Read the model definition and answer for the solid it produces. Units are mm, in the model's axes. Coordinates: 2 decimals unless noted, no trailing zeros. Order: outer loops, then holes, each group sorted by start corner. A loop starts at its lowest first (then second) coordinate and runs counter-clockwise, first axis right, second up. Notation, with made-up numbers: (-8, -12) -> (20, -12) arc R22 ccw to (20, 11) -> close; hole circle Ø2 at (83, 38). An arc over 180 degrees is marked (long way). Answer as a JSON object with one key per item and string values. Group by question number.
1) Given pin 1 (5.5 mm diameter, centred on y = 0, z = -48, fed in from +X); pin 2 (2 mm diameter, centred on x = 6.5, z = 40.5, fed in from -Y), each flat-ended and moving along its own axis, determine where each tip first touches the part or whether it passes through.
2) Consider L1, parallel to Z at x = 2.9, y = 0; L2, parallel to Z at x = 5.5, y = 0; L3, parallel to Y at x = 3.85, z = 0. Determine where each line is inside the solid, lowest interval first.
3) Section D-D on x = 8 is taken. Determine the outline of the cut face in (y, z).
4) Section C-C on y = 15 is taken. Determine the outline of the cut face in (x, z).
5) Section B-B on z = -24 is taken. Determine the outline of the cut face in (x, y), and give its area (3 significant figures).
6) Section A-A on y = 0 is taken. Determine the outline of the cut face in (x, z).
from build123d import *

# Parameters (mm, degrees)
F0_W            = 10
F0_H            = 17
F2_R            = 3.5
F3_DEPTH        = 10.001
F3_COPIES_COUNT = 6
F5_DEPTH        = 10.001
F6_R            = 39.5
F6_R_2          = 37
F7_DEPTH        = 5


# Not quite as in the source:
# - a pattern or mirror of a feature is missing from the dataset's text; its kind, count and spacing are read off the source's solid


with BuildPart() as f1:
    # F0 (on Front) → F1 (revolve)
    with BuildSketch(Plane.XZ):
        with Locations((5, 45.5)):
            Rectangle(F0_W, F0_H)
    revolve(axis=Axis((-28.7704151153, 0, 0), (-1, 0, 0)))

    # F2 (on face) → F3 (cut, through all)
    with BuildSketch(Plane(origin=(0, 0, 0), x_dir=(0, -1, 0), z_dir=(-1, 0, 0))):
        with Locations((41.5692193817, 24)):
            Circle(F2_R)
    f3 = extrude(amount=-F3_DEPTH, mode=Mode.SUBTRACT)

    # F3_copies: F3 ×6 about axis
    f3_copies_axis = Axis((0, 0, 0), (1, 0, 0))
    for i in range(1, F3_COPIES_COUNT):
        add(f3.rotate(f3_copies_axis, i * 360 / F3_COPIES_COUNT), mode=Mode.SUBTRACT)

    # F4 (on face) → F5 (cut, through all)
    with BuildSketch(Plane(origin=(0, 0, 0), x_dir=(0, -1, 0), z_dir=(-1, 0, 0))):
        with BuildLine():
            Line((-50, -20.3960780544), (-50, 20.3960780544))
            ThreePointArc((-50, 20.3960780544), (-54, 0), (-50, -20.3960780544))
        make_face()
        with BuildLine():
            ThreePointArc((54, 0), (52.990565198, 10.3923048454), (50, 20.3960780544))
            Line((50, 20.3960780544), (50, -20.3960780544))
            ThreePointArc((50, -20.3960780544), (52.990565198, -10.3923048454), (54, 0))
        make_face()
    extrude(amount=-F5_DEPTH, mode=Mode.SUBTRACT)

    # F6 (on face) → F7 (cut)
    with BuildSketch(Plane.YZ.offset(10)):
        Circle(F6_R)
        Circle(F6_R_2, mode=Mode.SUBTRACT)
    extrude(amount=-F7_DEPTH, mode=Mode.SUBTRACT)


solid = f1.part
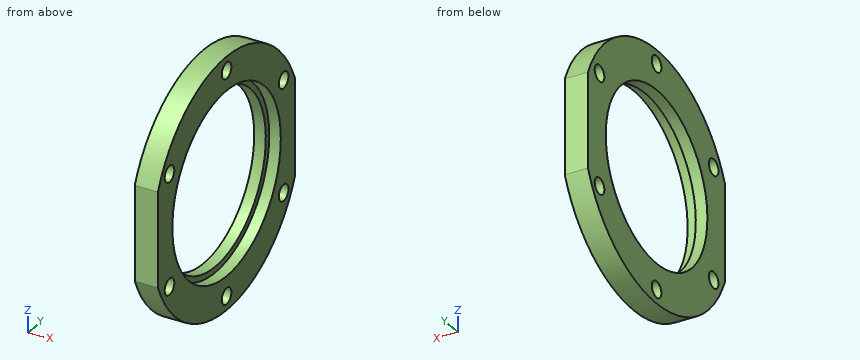
Worked answers:
{
 "1": {"pin 1": "passes through", "pin 2": "stops at y = -36.82"},
 "2": {"L1": "z = -54 to -51.5, -44.5 to -37, 37 to 44.5, 51.5 to 54", "L2": "z = -54 to -51.5, -44.5 to -39.5, 39.5 to 44.5, 51.5 to 54", "L3": "y = -50 to -37, 37 to 50"},
 "3": {"outline": "(-50, -20.4) arc R54 ccw to (50, -20.4) -> (50, 20.4) arc R54 ccw to (-50, 20.4) -> close; hole circle Ø7 at (-41.57, -24); hole circle Ø7 at (-41.57, 24); hole circle Ø79 at (0, 0); hole circle Ø7 at (0, -48); hole circle Ø7 at (0, 48); hole circle Ø7 at (41.57, -24); hole circle Ø7 at (41.57, 24)"},
 "4": {"outline": "(0, -51.87) -> (10, -51.87) -> (10, -36.54) -> (5, -36.54) -> (5, -33.82) -> (0, -33.82) -> close; (0, 33.82) -> (5, 33.82) -> (5, 36.54) -> (10, 36.54) -> (10, 51.87) -> (0, 51.87) -> close"},
 "5": {"outline": "(0, -48.37) -> (10, -48.37) -> (10, -45.07) -> (0, -45.07) -> close; (0, -38.07) -> (10, -38.07) -> (10, -31.37) -> (5, -31.37) -> (5, -28.16) -> (0, -28.16) -> close; (0, 28.16) -> (5, 28.16) -> (5, 31.37) -> (10, 31.37) -> (10, 38.07) -> (0, 38.07) -> close; (0, 45.07) -> (10, 45.07) -> (10, 48.37) -> (0, 48.37) -> close", "area": "232 mm²"},
 "6": {"outline": "(0, -54) -> (10, -54) -> (10, -51.5) -> (0, -51.5) -> close; (0, -44.5) -> (10, -44.5) -> (10, -39.5) -> (5, -39.5) -> (5, -37) -> (0, -37) -> close; (0, 37) -> (5, 37) -> (5, 39.5) -> (10, 39.5) -> (10, 44.5) -> (0, 44.5) -> close; (0, 51.5) -> (10, 51.5) -> (10, 54) -> (0, 54) -> close"}
}
